Check sheet for the drawn part. Datum: minimum x, y, z corner. Units: mm. Coordinates: 2 decimals unless noted, no trailing zeros. Order: outer loops, then holes, each group sorted by start corner. A loop starts at its lowest first (then second) coordinate and runs counter-clockwise, first axis right, second up. Notation, with made-up numbers: M 73,60 L 121,60 A22 ccw 121,89 Z; hole C -26.75,-7.5 d2. An arc over 180 degrees is marked long. Use one line per item in the form item = value. Start each with the question number.
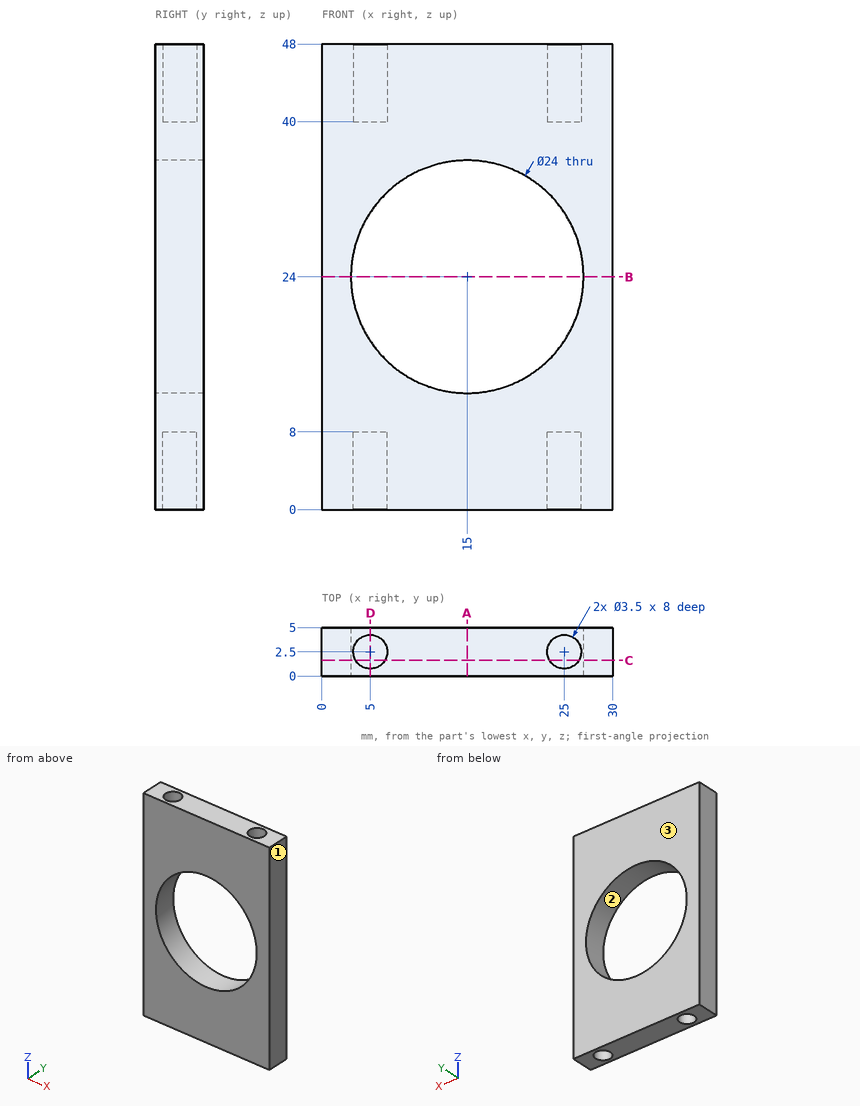
1. Cross-section at B-B on z = 24. Enter the section's corners in (x, y).
2. Release check for a two-part mould opening along X. For the marked faces 1, 2 and 3 record: pulls with the +X half, pulls with the -X half, needs draft (parallel to the pull), parting line crosses it, or undercut.
3. Depth check by flat-ended pin: P1, Ø1, axis at x = 5, y = 2.5, coming from the +Z side; P2, Ø1.8, axis at x = 5, y = 2, coming from the -Z side. Enter the tip coordinate at first touch or a pass-through.
4. Material ranges on line 1 along X through (y, z) = (2.5, 46.5); line 2 along Y through (x, z) = (25, 4); line 3 along X through (y, z) = (1.4, 45.5), recorded low to high.
5. Cross-section at A-A on x = 15. Enter the section's corners in (y, z).
6. Cross-section at C-C on y = 1.6. Enter the section's corners in (x, z).
7. Cross-section at D-D on x = 5. Enter the section's corners in (y, z).
Final values:
q1.outline = M 0,0 L 3,0 L 3,5 L 0,5 Z; M 27,0 L 30,0 L 30,5 L 27,5 Z
q2.face_1 = pulls with the +X half
q2.face_2 = undercut
q2.face_3 = needs draft
q3.P1 = 40
q3.P2 = 8
q4.line_1 = 0 to 3.25, 6.75 to 23.25, 26.75 to 30
q4.line_2 = 0 to 0.75, 4.25 to 5
q4.line_3 = 0 to 3.64, 6.36 to 23.64, 26.36 to 30
q5.outline = M 0,0 L 5,0 L 5,12 L 0,12 Z; M 0,36 L 5,36 L 5,48 L 0,48 Z
q6.outline = M 0,0 L 3.5,0 L 3.5,8 L 6.5,8 L 6.5,0 L 23.5,0 L 23.5,8 L 26.5,8 L 26.5,0 L 30,0 L 30,48 L 26.5,48 L 26.5,40 L 23.5,40 L 23.5,48 L 6.5,48 L 6.5,40 L 3.5,40 L 3.5,48 L 0,48 Z; hole C 15,24 d24
q7.outline = M 0,0 L 0.75,0 L 0.75,8 L 4.25,8 L 4.25,0 L 5,0 L 5,17.37 L 0,17.37 Z; M 0,30.63 L 5,30.63 L 5,48 L 4.25,48 L 4.25,40 L 0.75,40 L 0.75,48 L 0,48 Z
